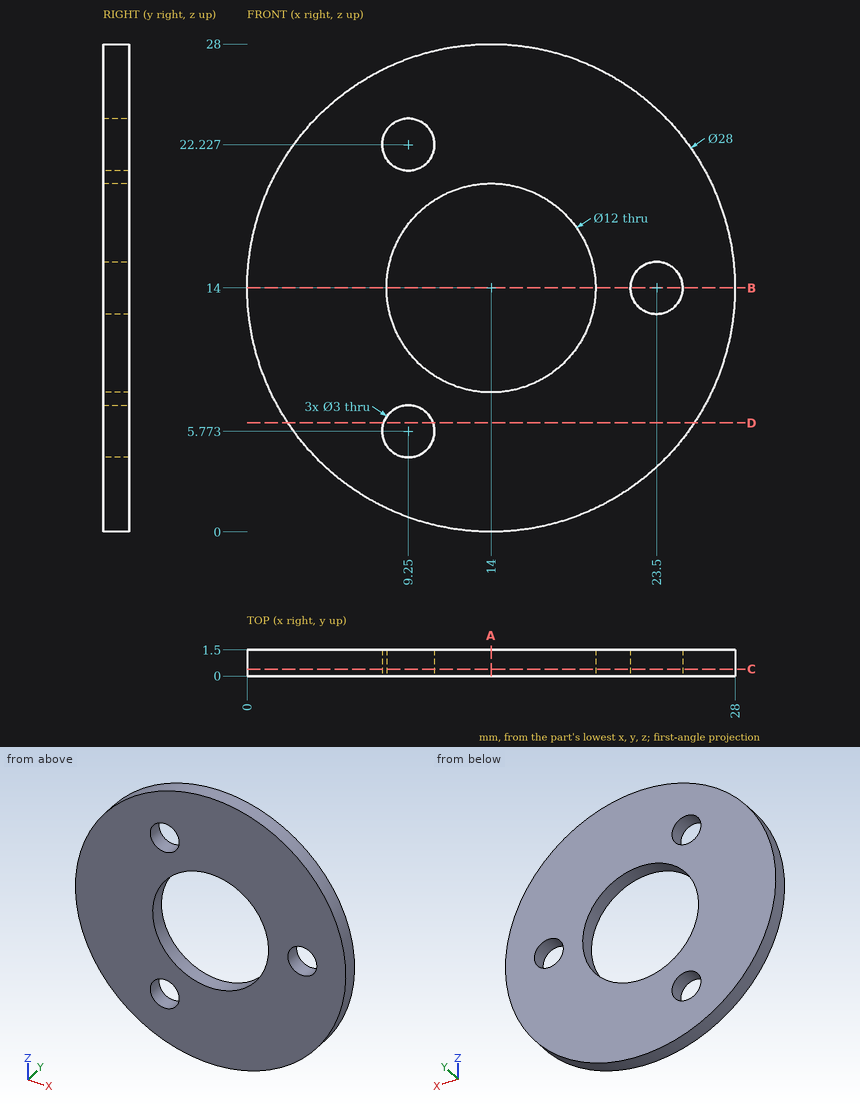
The figure shows three views and two pictorial views of one solid part (mm, origin at its lowest corner). Answer the questions. Coordinates: 2 decimals unless noted, no trailing zeros. Order: outer loops, then holes, each group sorted by start corner. A loop starts at its lowest first (then second) coordinate and runs counter-clockwise, first axis right, second up.
Q1. Given P1, Ø11, axis at x = 14, z = 14, coming from the -Y side, flat-ended and moving along its own axis, determine where the tip first touches the part or whether it passes through.
Q2. A cutting plane is placed at A-A, the plane x = 14. Write down the section's boundary in (y, z), and give its area (3 significant figures).
Q3. A cutting plane is placed at D-D, the plane z = 6.25. Write down the section's boundary in (x, y), and give its area (3 significant figures).
Q4. A cutting plane is placed at B-B, the plane z = 14. Write down the section's boundary in (x, y), and give its area (3 significant figures).
Q5. A cutting plane is placed at C-C, the plane y = 0.4. Write down the section's boundary in (x, z).
Q6. Consider line 1 (X direction, y = 0.45, z = 14); line 2 (Z direction, x = 9.25, y = 0.45) (1 decimal); line 3 (X direction, y = 0.6, z = 6.5). Determine where each line is inside the solid, lowest interval first.
Answers follow:
1. P1: passes through
2. outline: (0, 0) - (1.5, 0) - (1.5, 8) - (0, 8) - close; (0, 20) - (1.5, 20) - (1.5, 28) - (0, 28) - close
2. area: 24.0 mm2
3. outline: (2.34, 0) - (7.83, 0) - (7.83, 1.5) - (2.34, 1.5) - close; (10.67, 0) - (25.66, 0) - (25.66, 1.5) - (10.67, 1.5) - close
3. area: 30.7 mm2
4. outline: (0, 0) - (8, 0) - (8, 1.5) - (0, 1.5) - close; (20, 0) - (22, 0) - (22, 1.5) - (20, 1.5) - close; (25, 0) - (28, 0) - (28, 1.5) - (25, 1.5) - close
4. area: 19.5 mm2
5. outline: circle Ø28 at (14, 14); hole circle Ø3 at (9.25, 5.77); hole circle Ø3 at (9.25, 22.23); hole circle Ø12 at (14, 14); hole circle Ø3 at (23.5, 14)
6. line 1: x = 0 to 8, 20 to 22, 25 to 28
6. line 2: z = 0.8 to 4.3, 7.3 to 10.3, 17.7 to 20.7, 23.7 to 27.2
6. line 3: x = 2.18 to 7.94, 10.56 to 25.82
